from build123d import *

# Parameters (mm, degrees)
F0_W     = 228.6
F0_H     = 38.1
F1_DEPTH = 2.65684
F2_W     = 228.6
F2_H     = 38.1
F3_DEPTH = 2.65684
F4_R     = 3.96875
F5_DEPTH = 2.65684
F6_R     = 4.365625
F7_DEPTH = 2.65684
F8_R     = 2.54
F9_R     = 1.27


# Not quite as in the source:
# - a pattern or mirror of a feature is missing from the dataset's text; its kind, count and spacing are read off the source's solid


with BuildPart() as f1:
    # F0 (on Front) → F1 (new body)
    with BuildSketch(Plane.XZ):
        Rectangle(F0_W, F0_H)
    extrude(amount=F1_DEPTH)

    # F2 (on face) → F3 (join)
    with BuildSketch(Plane(origin=(0, 0, -19.05), x_dir=(1, 0, 0), z_dir=(0, 0, -1))):
        with Locations((0, 19.05)):
            Rectangle(F2_W, F2_H)
    extrude(amount=-F3_DEPTH)

    # F4 (on face) → F5 (cut)
    with BuildSketch(Plane.XZ.offset(2.65684)):
        with Locations((-45.72, 6.35)):
            Circle(F4_R)
        with Locations((-57.15, -3.175)):
            Circle(F4_R)
    f5 = extrude(amount=-F5_DEPTH, mode=Mode.SUBTRACT)

    # F5_copies: F5 across plane
    add(f5.mirror(Plane(origin=(0, 0, 0), x_dir=(0, 0, 1), z_dir=(1, 0, 0))), mode=Mode.SUBTRACT)

    # F6 (on face) → F7 (cut)
    with BuildSketch(Plane(origin=(0, 0, -19.05), x_dir=(1, 0, 0), z_dir=(0, 0, -1))):
        with Locations((-91.44, 22.86)):
            Circle(F6_R)
        with Locations((0, 22.86)):
            Circle(F6_R)
        with Locations((91.44, 22.86)):
            Circle(F6_R)
    extrude(amount=-F7_DEPTH, mode=Mode.SUBTRACT)

    # F8
    f8_edges = [f1.edges().sort_by_distance(p)[0] for p in [
        (0, 0, -19.05),
    ]]
    fillet(f8_edges, radius=F8_R)

    # F9
    f9_edges = [f1.edges().sort_by_distance(p)[0] for p in [
        (0, -2.65684, -16.39316),
    ]]
    fillet(f9_edges, radius=F9_R)


solid = f1.part
Could you check a few things on this model? Use its own coordinates, in mm. A direction names the side the tool comes from. Coordinates: 2 decimals unless noted, no trailing zeros. Write each loop counter-clockwise with the first axis right and the second up, starting at its lowest first coordinate (ties: lowest second). Pieces come first, ordered by that corner, then holes. Notation, with made-up numbers: (-12, -4.75) - (40, -4.75) arc R14 cw to (40, 19.25) - close; hole circle Ø4 at (-18.5, 78.25). An arc over 180 degrees is marked (long way). Put each result on its own line as item: value. Start each with the question number.
Q1. Thinking about a two-plate mould opening in Z: for faces 3 (the cylindrical face through (61.115, -1.347, -3.001)), 4 (the cylindrical face through (-61.115, -1.347, -3.001)), 5 (the flat face through (-2, -16, -19.05)), 6 (the cylindrical face through (93.79, -26.54, -17.74)), which applies, pulls with the +Z half, pulls with the -Z half, needs draft (parallel to the pull), parting line crosses it, or undercut?
Q2. I want a section at B-B on x = 91.44. Write out the boundary of the cut face in (y, z).
Q3. I want a section at D-D on y = -8. Write out the boundary of the cut face in (x, z), plus the area to 3 significant figures.
Q4. I'm going to push flat-ended pins straight in: P1, Ø10.5, axis at x = 36.5, z = 5.5, coming from the -Y side; P2, Ø17, axis at x = 56.5, y = -26.5, coming from the +Z side. Where does each tip first touch, or does it pass through?
Q5. I want a section at A-A on z = 6.35. Write out the boundary of the cut face in (x, y).
Q6. I want a section at C-C on x = 16. Write out the boundary of the cut face in (y, z).
Q7. Please list where these lines run through material, in increasing order: L1, parallel to X at y = -22.86, z = -17.25; L2, parallel to X at y = -1, z = 6; L3, parallel to Z at x = -57.15, y = -1.
Q8. Which directions (+Z, -Z, +X, -X, +Y, -Y) give clear straight access to the entire face, cutting with the end or side of a thin tool? Please do faces 1 (the flat face through (-2, -17, -16.393)), 2 (the cylindrical face through (-95.8, -23.1, -17.7)).
Checks:
1. face 3: undercut
1. face 4: undercut
1. face 5: pulls with the -Z half
1. face 6: needs draft
2. outline: (-38.1, -19.05) - (-27.23, -19.05) - (-27.23, -16.39) - (-38.1, -16.39) - close; (-18.49, -19.05) - (-2.54, -19.05) arc R2.54 ccw to (0, -16.51) - (0, 19.05) - (-2.66, 19.05) - (-2.66, -15.12) arc R1.27 cw to (-3.93, -16.39) - (-18.49, -16.39) - close
3. outline: (-114.3, -19.05) - (114.3, -19.05) - (114.3, -16.39) - (-114.3, -16.39) - close
3. area: 607 mm²
4. P1: y = -2.66
4. P2: z = -16.39
5. outline: (-114.3, -2.66) - (-49.69, -2.66) - (-49.69, 0) - (-114.3, 0) - close; (-41.75, -2.66) - (41.75, -2.66) - (41.75, 0) - (-41.75, 0) - close; (49.69, -2.66) - (114.3, -2.66) - (114.3, 0) - (49.69, 0) - close
6. outline: (-38.1, -19.05) - (-2.54, -19.05) arc R2.54 ccw to (0, -16.51) - (0, 19.05) - (-2.66, 19.05) - (-2.66, -15.12) arc R1.27 cw to (-3.93, -16.39) - (-38.1, -16.39) - close
7. L1: -114.3 to -95.81, -87.07 to -4.37, 4.37 to 87.07, 95.81 to 114.3
7. L2: -114.3 to -49.67, -41.77 to 41.77, 49.67 to 114.3
7. L3: -18.53 to -7.14, 0.79 to 19.05
8. face 1: +Z, +X, -X, -Y
8. face 2: +Z, -Z
